from build123d import *

# Parameters (mm, degrees)
F0_W        = 127
F0_H        = 76.2
F0_R        = 6.0082051914
F0_R_2      = 6.35
F1_DEPTH    = 50.8
F2_R        = 5.0727698676
F3_DEPTH    = 72.136
F4_T1_DEPTH = 192.3207478943
F5_T1_DEPTH = 190.5
F6_T1_DEPTH = 57.15
F6_T3_DEPTH = 95.25
F6_T6_ANGLE = 90.000000001
F6_T8_ANGLE = 90.000000001


# Not quite as in the source:
# - a fillet or chamfer that OpenCascade refuses, or shapes differently, is made with other operations: its cross-section is extruded or revolved along the edge and cut away or added


with BuildPart() as f1:
    # F0 (on Front) → F1 (new body)
    with BuildSketch(Plane.XZ):
        with Locations((-14.6853402257, 47.3040914883)):
            Rectangle(F0_W, F0_H)
        with Locations((-60.8313269913, 73.5488906503)):
            Circle(F0_R, mode=Mode.SUBTRACT)
        with Locations((29.7646597743, 60.0040914883)):
            Circle(F0_R_2, mode=Mode.SUBTRACT)
    extrude(amount=F1_DEPTH)

    # F2 (on face) → F3 (cut)
    with BuildSketch(Plane.XZ.offset(50.8)):
        with Locations((0, 46.5039759874)):
            Circle(F2_R)
    extrude(amount=-F3_DEPTH, mode=Mode.SUBTRACT)

    # F4: chamfer of 12.7 on 1 edges, made by hand

    # F4_s2 → F4_t1 (cut)
    with BuildSketch(Plane.YZ.offset(-110.8457141729)):
        Polygon((-38.1, 85.4040914883), (-50.8, 72.7040914883), (-50.8, 85.4040914883), align=None)
    extrude(amount=F4_T1_DEPTH, mode=Mode.SUBTRACT)

    # F5: fillet of radius 12.7 on 1 edges, made by hand

    # F5_s2 → F5_t1 (cut)
    with BuildSketch(Plane.YZ.offset(-109.9353402257)):
        with BuildLine():
            ThreePointArc((0, 72.7040914883), (-3.7197438789, 81.6843476094), (-12.7, 85.4040914883))
            Line((-12.7, 85.4040914883), (0, 85.4040914883))
            Line((0, 85.4040914883), (0, 72.7040914883))
        make_face()
    extrude(amount=F5_T1_DEPTH, mode=Mode.SUBTRACT)

    # F6: fillet of radius 12.7 on 2 edges, made by hand

    # F6_s2 → F6_t1 (cut)
    with BuildSketch(Plane.XZ.offset(12.7)):
        with BuildLine():
            ThreePointArc((-65.4853402257, 85.4040914883), (-74.4655963468, 81.6843476094), (-78.1853402257, 72.7040914883))
            Line((-78.1853402257, 72.7040914883), (-78.1853402257, 85.4040914883))
            Line((-78.1853402257, 85.4040914883), (-65.4853402257, 85.4040914883))
        make_face()
        with BuildLine():
            ThreePointArc((48.8146597743, 72.7040914883), (45.0949158954, 81.6843476094), (36.1146597743, 85.4040914883))
            Line((36.1146597743, 85.4040914883), (48.8146597743, 85.4040914883))
            Line((48.8146597743, 85.4040914883), (48.8146597743, 72.7040914883))
        make_face()
    extrude(amount=F6_T1_DEPTH, mode=Mode.SUBTRACT)

    # F6_s4 → F6_t3 (cut)
    with BuildSketch(Plane.XY.offset(-22.5459085117)):
        with BuildLine():
            ThreePointArc((48.8146597743, -12.7), (45.0949158954, -3.7197438789), (36.1146597743, 0))
            Line((36.1146597743, 0), (48.8146597743, 0))
            Line((48.8146597743, 0), (48.8146597743, -12.7))
        make_face()
        with BuildLine():
            ThreePointArc((-65.4853402257, 0), (-74.4655963468, -3.7197438789), (-78.1853402257, -12.7))
            Line((-78.1853402257, -12.7), (-78.1853402257, 0))
            Line((-78.1853402257, 0), (-65.4853402257, 0))
        make_face()
    extrude(amount=F6_T3_DEPTH, mode=Mode.SUBTRACT)

    # F6_s5 → F6_t6 (revolve, cut)
    with BuildSketch(Plane.XZ.offset(12.6999999999)):
        with BuildLine():
            ThreePointArc((48.8146597743, 72.7040914883), (45.0949158954, 81.6843476094), (36.1146597743, 85.4040914883))
            Line((36.1146597743, 85.4040914883), (48.8146597743, 85.4040914883))
            Line((48.8146597743, 85.4040914883), (48.8146597743, 72.7040914883))
        make_face()
    revolve(axis=Axis((48.8146597743, -12.6999999999, 72.7040914884), (-1, 0, 0)), revolution_arc=F6_T6_ANGLE, mode=Mode.SUBTRACT)

    # F6_s7 → F6_t8 (revolve, cut)
    with BuildSketch(Plane.XZ.offset(12.6999999999)):
        with BuildLine():
            ThreePointArc((-65.4853402257, 85.4040914883), (-74.4655963468, 81.6843476094), (-78.1853402257, 72.7040914883))
            Line((-78.1853402257, 72.7040914883), (-78.1853402257, 85.4040914883))
            Line((-78.1853402257, 85.4040914883), (-65.4853402257, 85.4040914883))
        make_face()
    revolve(axis=Axis((-78.1853402257, -12.6999999999, 72.7040914884), (-1, 0, 0)), revolution_arc=F6_T8_ANGLE, mode=Mode.SUBTRACT)


solid = f1.part
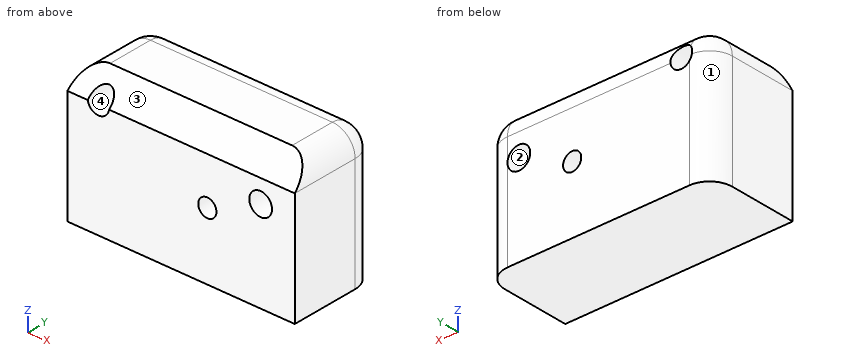
Source: CAD feature listing. Evaluate the final solid. Frame: model axes, mm. Face numbers are marked on the shaded views. Round coordinates to 2 decimals unless told otherwise and drop trailing zeros. Loops run counter-clockwise (first coordinate to the right, second up) from the corner with the lowest first, then second, coordinate; pieces in that order, holes last. Notation, with made-up numbers: M 14,27 L 27,27 A17 cw 27,59 Z; hole C 86,34.25 d3. An arc over 180 degrees is marked long. Return JSON: item names as keys, results as strings. Group by question number.
1. Section query B-B on y = -7.5. Output: boundary loops of the cut face in (x, z), and give its area (3 significant figures).
2. Section query A-A on x = 0. Output: boundary loops of the cut face in (y, z), and give its area (3 significant figures).
3. Section query D-D on y = -43. Output: boundary loops of the cut face in (x, z), and give its area (3 significant figures).
4. Mould query, pull axis Z, two halves, no side actions, for the marked faces 1, 2, 3 and 4. Classes: released by +Z, released by -Z, zero draft, split by the parting line, or undercut.
5. Pin query (flat end, axial travel): pin 1 (12 mm diameter, centred on x = 32, z = 49.5, fed in from +Y). Return the tip coordinate at first contact, or that it passes through.
6. Section query C-C on x = 22. Output: boundary loops of the cut face in (y, z), and give its area (3 significant figures).
7. Material intervals for line 1 along Z through (x, y) = (0, -28); line 2 along Z through (x, y) = (35, -40); line 3 along X through (y, z) = (-32, 43.5), sorted ascending. Write a range as from..to.
Checks:
{
 "1": {"outline": "M -77.07,9.2 L 47.7,9.2 L 47.7,72.7 A11.59 ccw 36.11,84.29 L -65.49,84.29 A11.59 ccw -77.07,72.7 Z; hole C -60.83,73.55 d12.02; hole C 0,46.5 d10.15; hole C 29.76,60 d12.7", "area": "8,990 mm²"},
 "2": {"outline": "M -50.8,9.2 L 0,9.2 L 0,41.43 L -50.8,41.43 Z; M -50.8,51.58 L 0,51.58 L 0,72.7 A12.7 ccw -12.7,85.4 L -38.1,85.4 L -50.8,72.7 Z", "area": "3,240 mm²"},
 "3": {"outline": "M -78.19,9.2 L 48.81,9.2 L 48.81,72.7 A12.7 ccw 46.14,80.5 L -75.51,80.5 A12.7 ccw -78.19,72.7 Z; hole C -60.83,73.55 d12.02; hole C 0,46.5 d10.15; hole C 29.76,60 d12.7", "area": "8,720 mm²"},
 "4": {"face 1": "zero draft", "face 2": "undercut", "face 3": "released by +Z", "face 4": "undercut"},
 "5": {"pin 1": "stops at y = 0"},
 "6": {"outline": "M -50.8,9.2 L 0,9.2 L 0,72.7 A12.7 ccw -12.7,85.4 L -38.1,85.4 L -50.8,72.7 Z", "area": "3,760 mm²"},
 "7": {"line 1": "z = 9.2..41.43, 51.58..85.4", "line 2": "z = 9.2..56.41, 63.6..83.5", "line 3": "x = -78.19..-4.09, 4.09..48.81"}
}
